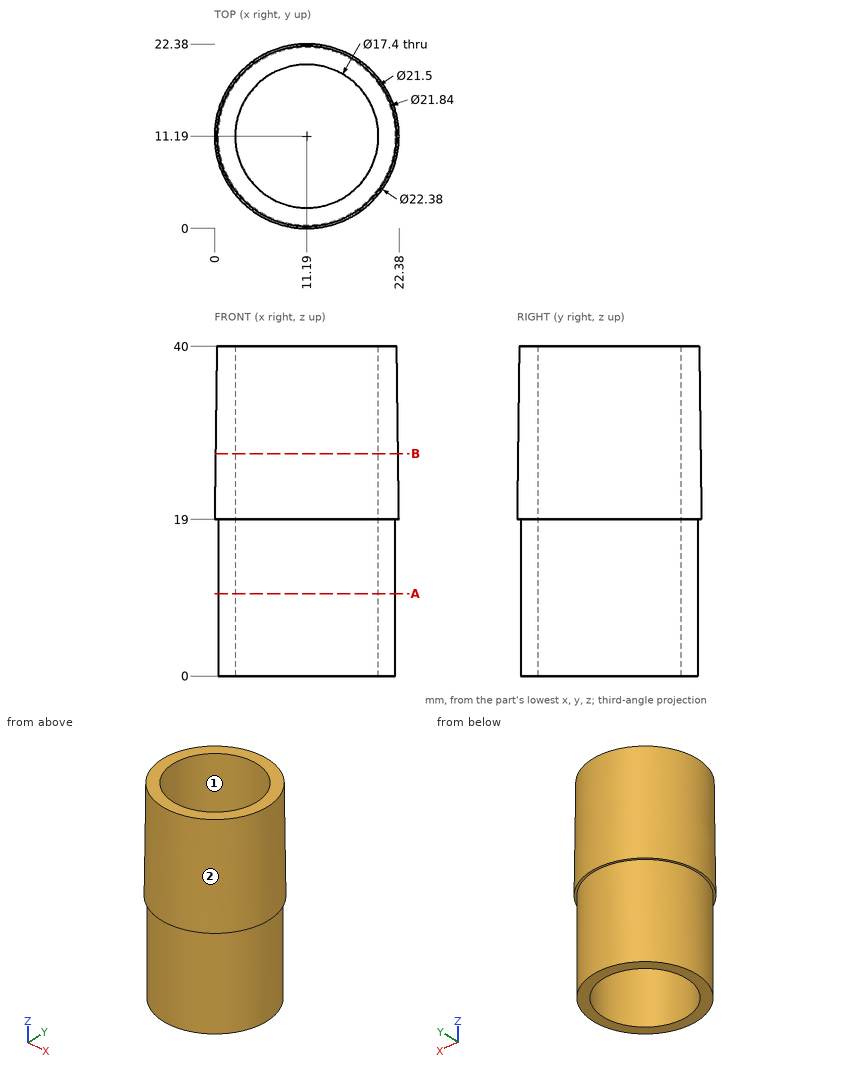
Geometry: see drawing. Coordinates: mm, zero at the bounding-box minimum. Give positions to 0.01 mm unless a question says otherwise; leave off trailing zeros. Write each loop counter-clockwise with the first axis right and the second up, starting at its lowest first coordinate (ties: lowest second). Pieces come first, ordered by that corner, then holes. Notation, with made-up numbers: (-31, 26) - (-5, 26) arc R30 cw to (-5, 64) - close; hole circle Ø1 at (-12, -11.75). An arc over 180 degrees is marked (long way). Return JSON: item names as keys, results as strings. Group by question number.
1) Line query: line 1 (Y direction, x = 11.19, z = 12); line 2 (X direction, y = 16.5, z = 25); line 3 (Y direction, x = 10, z = 20). Output: solid intervals per line, ascending.
2) Section A-A on z = 10. Return the cut outline in (x, y), plus the area to 3 significant figures.
3) Section B-B on z = 27. Return the cut outline in (x, y), plus the area to 3 significant figures.
4) Mould query, pull axis Y, two halves, no side actions, for the marked faces 1 and 2. Classes: released by +Y, released by -Y, zero draft, split by the parting line, or undercut.
5) First-contact query: P1, Ø1, axis at x = 2.5, z = 24.5, coming from the -Y side; P2, Ø10, axis at x = 10, z = 10.5, coming from the -Y side; P3, Ø3, axis at x = 17.5, z = 8, coming from the +Y side. Flat tips, straight axial feed; report the tip coordinate or a pass-through.
Filled in:
{
 "1": {"line 1": "y = 0.44 to 2.49, 19.89 to 21.94", "line 2": "x = 1.43 to 4.3, 18.08 to 20.95", "line 3": "y = 0.08 to 2.57, 19.81 to 22.3"},
 "2": {"outline": "circle Ø21.5 at (11.19, 11.19); hole circle Ø17.4 at (11.19, 11.19)", "area": "125 mm^2"},
 "3": {"outline": "circle Ø22.17 at (11.19, 11.19); hole circle Ø17.4 at (11.19, 11.19)", "area": "148 mm^2"},
 "4": {"face 1": "undercut", "face 2": "split by the parting line"},
 "5": {"P1": "stops at y = 3.67", "P2": "stops at y = 0.44", "P3": "stops at y = 20.8"}
}
